Autodesk Inventor part; units mm, degrees
ref_plane "YZ Plane" through (0, 0, 0) normal (1, 0, 0) x (0, 1, 0)
ref_plane "XZ Plane" through (0, 0, 0) normal (0, 1, 0) x (-1, 0, 0)
ref_plane "XY Plane" through (0, 0, 0) normal (0, 0, 1) x (1, 0, 0)
sketch "Sketch1" plane through (0, 0, 0) normal (0, 0, 1) x (1, 0, 0)
  line L0 (0, 0) -> (0, 13.4062) construction
  line L1 (0, 0) -> (20.3742, 0) construction
  circle A0 centre (9.525, 12.7) radius 9.525 construction
  circle A1 centre (9.525, 12.7) radius 3.2004
  arc A2 (3.3908, 14.3415) -> (7.8407, 6.5775) centre (9.525, 12.7) ccw
  line L2 (31.75, 0) -> (76.2, 0)
  line L3 (76.2, 0) -> (76.2, 25.4)
  line L4 (76.2, 25.4) -> (31.75, 25.4)
  line L5 (31.75, 25.4) -> (31.75, 31.75)
  line L6 (31.75, 31.75) -> (31.75, 31.75)
  line L7 (31.75, 31.75) -> (31.75, 69.85)
  line L8 (31.75, 69.85) -> (6.35, 69.85)
  line L9 (6.35, 69.85) -> (6.35, 25.4)
  line L10 (6.35, 25.4) -> (3.3908, 14.3415)
  circle A3 centre (19.05, 63.5) radius 2.4892
  circle A4 centre (19.05, 50.8) radius 2.4892
  circle A5 centre (19.05, 38.1) radius 2.4892
  circle A6 centre (44.45, 12.7) radius 2.4892
  circle A7 centre (57.15, 12.7) radius 2.4892
  circle A8 centre (69.85, 12.7) radius 2.4892
  line L11 (31.75, 31.75) -> (31.75, 25.4)
  line L12 (31.75, 25.4) -> (31.75, 25.4)
  line L13 (31.75, 0) -> (7.8407, 6.5775)
  arc A9 (67.9888, -8.047) -> (76.2, -4.7625) centre (71.4375, -4.7625) ccw
  circle A10 centre (71.4375, -4.7625) radius 2.4892
  line L14 (76.2, -4.7625) -> (76.2, 0)
  line L15 (67.9888, -8.047) -> (60.325, 0)
  arc A11 (31.75, 29.8901) -> (36.2401, 25.4) centre (33.9951, 27.6451) ccw
  circle A12 centre (31.2871, 27.4957) radius 0.4629 construction
  circle A13 centre (33.8457, 24.9371) radius 0.4629 construction
  line L16 (31.2871, 27.4957) -> (31.75, 25.4) construction
  line L17 (31.75, 25.4) -> (33.8457, 24.9371) construction
  point P0 (76.2, 12.7)
  point P1 (19.05, 69.85)
  dimension "d0" = 19.05
  dimension "d2" = 6.4008
  dimension "d6" = 12.7
  dimension "d7" = 25.4
  dimension "d8" = 4.9784
  dimension "d11" = 12.7
  dimension "d16" = 6.35
  dimension "d17" = 25.4
  dimension "d19" = 6.35
  dimension "d20" = 12.7
  dimension "d21" = 6.35
  dimension "d24" = 12.7
  dimension "d29" = 6.35
  dimension "d30" = 12.7
  dimension "d35" = 25.4
  dimension "d36" = 9.525
  dimension "d37" = 4.9784
  dimension "d38" = 3.175
  dimension "d39" = 15.875
  dimension "d40" = 6.35
extrude "Extrusion1" add sketch "Sketch1" along normal blind 3.175 contours L10 L9 L8 L7 L5 A11 L4 L3 L2 L13 A2 | L2 L14 A9 L15
fillet "Fillet1" radius 3.175 6 edges at (6.35, 69.85, 1.5875) (31.75, 69.85, 1.5875) (76.2, 25.4, 1.5875) (6.35, 25.4, 1.5875) (31.75, 0, 1.5875) (60.325, 0, 1.5875)
equation "\"d24\" = d11"
properties part number "Bottom Bearing Plate Final (R4A - 0.25in Between Stages)" material "Aluminum 6061"
Geometry check sheet. Reference: the model listing, model coordinates, mm. A direction names the side the tool comes from. Coordinates: 2 decimals unless noted, no trailing zeros. Order: outer loops, then holes, each group sorted by start corner. A loop starts at its lowest first (then second) coordinate and runs counter-clockwise, first axis right, second up. Notation, with made-up numbers: (-30, 60) - (-11, 60) arc R37 cw to (-11, 97) - close; hole circle Ø4 at (60, 43.5). An arc over 180 degrees is marked (long way). Answer in a Markdown table with one row per item. Add a question column.
1. Section check A-A (y = 63.5). Enter the section's corners in (x, z) (3 decimals).
2. Section check B-B (x = 44.45). Enter the section's corners in (y, z) (3 decimals), plus the area to 3 significant figures.
3. Section check C-C (z = 0.9). Give the number of separate pieces and of enclosed holes in the cut face, plus the area to 3 significant figures.
4. Material ranges on L1, parallel to Y at x = 19.05, z = 0.9; L2, parallel to Y at x = 69.85, z = 1.15; L3, parallel to Y at x = 44.45, z = 0.95, recorded low to high. Write a range as [from, to].
5. Gauge pin test, flat ends, axial feed: pin 1 Ø1.6 at (x, z) = (41.5, 2.5) entering from -Y; pin 2 Ø4 at (x, y) = (71.44, -4.76) entering from +Z; pin 3 Ø8.5 at (x, y) = (9.525, 12.7) entering from -Z. Record the tip position at first contact, or that the pin passes through.
6. Section check D-D (y = 12.7). Enter the section's corners in (x, z) (3 decimals).
7. Draft check along Y on faces 1 (the face through (7.3, 68.94, 1.61)), 2 (the face through (18.51, 53.23, 1.57)), 3 (the face through (31, 31, 3.175)). Enter one of: +Y half, -Y half, draft (parallel to the pull), parting line (faces both ways), or undercut.
8. Access from +Z, -Z, +X, -X, +Y, -Y to the whole of each face (thin tool, end or side, straight path). Record for faces 4 (the face through (31.75, 48, 2)), 5 (the face through (68.95, -4.87, 1.57)).
Data:
| question | item | result |
|---|---|---|
| 1 | outline | (6.35, 0) - (16.561, 0) - (16.561, 3.175) - (6.35, 3.175) - close; (21.539, 0) - (31.75, 0) - (31.75, 3.175) - (21.539, 3.175) - close |
| 2 | outline | (0, 0) - (10.211, 0) - (10.211, 3.175) - (0, 3.175) - close; (15.189, 0) - (25.4, 0) - (25.4, 3.175) - (15.189, 3.175) - close |
| 2 | area | 64.8 mm² |
| 3 | separate pieces | 1 |
| 3 | enclosed holes | 8 |
| 3 | area | 2,770 mm² |
| 4 | L1 | y = [3.49, 35.61], [40.59, 48.31], [53.29, 61.01], [65.99, 69.85] |
| 4 | L2 | y = [-9.25, -6.68], [-2.85, 10.21], [15.19, 25.4] |
| 4 | L3 | y = [0, 10.21], [15.19, 25.4] |
| 5 | pin 1 | stops at y = 0 |
| 5 | pin 2 | passes through |
| 5 | pin 3 | stops at z = 0 |
| 6 | outline | (3.175, 0) - (6.325, 0) - (6.325, 3.175) - (3.175, 3.175) - close; (12.725, 0) - (41.961, 0) - (41.961, 3.175) - (12.725, 3.175) - close; (46.939, 0) - (54.661, 0) - (54.661, 3.175) - (46.939, 3.175) - close; (59.639, 0) - (67.361, 0) - (67.361, 3.175) - (59.639, 3.175) - close; (72.339, 0) - (76.2, 0) - (76.2, 3.175) - (72.339, 3.175) - close |
| 7 | face 1 | +Y half |
| 7 | face 2 | undercut |
| 7 | face 3 | draft |
| 8 | face 4 | +Z, -Z, +X, +Y |
| 8 | face 5 | +Z, -Z |
